Verification items for this drawing (mm, ordinates from the low corner). A direction names the side the tool comes from. Coordinates: 2 decimals unless noted, no trailing zeros. Write each loop counter-clockwise with the first axis right and the second up, starting at its lowest first coordinate (ties: lowest second). Pieces come first, ordered by that corner, then holes. Notation, with made-up numbers: M -34.5,88.25 L 10.5,88.25 A30 ccw 10.5,121.25 Z; hole C 54.25,41.5 d2. An arc over 180 degrees is marked long. Answer as CSV lines item,"result". Start each with the question number.
1) Section check D-D (x = 6). Record the cut outline in (y, z), and give its area (3 significant figures).
2) Draft check along X on the marked faces 1, 2 and 3. Enter one of: +X half, -X half, draft (parallel to the pull), parting line (faces both ways), or undercut.
3) Go/stop test with flat-tipped pins: pin 1 Ø1 at (x, z) = (12.5, 4) entering from -Y; pin 2 Ø3 at (y, z) = (17, 9.5) entering from -X; pin 3 Ø1.5 at (x, y) = (18, 25) entering from -Z (3 decimals). Record where each tip stops, or that it passes through.
4) Section check A-A (y = 19.05). Record the cut outline in (x, z) (1 decimal).
5) Material ranges on L1, parallel to Z at x = 22.5, y = 5; L2, parallel to X at y = 11, z = 2.5 (1 decimal); L3, parallel to X at y = 15, z = 8 (1 decimal), recorded low to high. Write a range as [from, to].
6) Access from +Z, -Z, +X, -X, +Y, -Y to the whole of each face (thin tool, end or side, straight path). Record for the marked faces 4, 5 and 6.
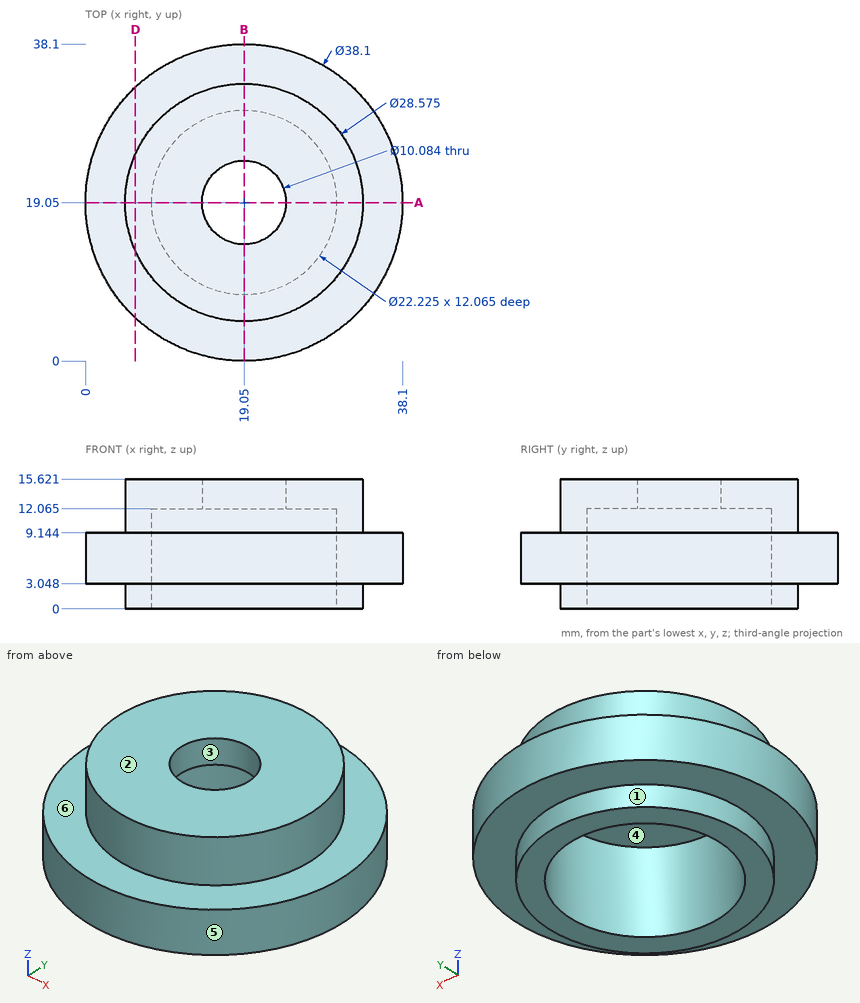
Results found:
1,outline,"M 5.17,3.05 L 13.23,3.05 L 13.23,0 L 24.87,0 L 24.87,3.05 L 32.93,3.05 L 32.93,9.14 L 24.87,9.14 L 24.87,15.62 L 13.23,15.62 L 13.23,9.14 L 5.17,9.14 Z"
1,area,"280 mm2"
2,face 1,"parting line"
2,face 2,"draft"
2,face 3,"undercut"
3,pin 1,"stops at y = 0.99"
3,pin 2,"stops at x = 0.01"
3,pin 3,"stops at z = 12.065"
4,outline,"M 0,3 L 4.8,3 L 4.8,0 L 7.9,0 L 7.9,12.1 L 14,12.1 L 14,15.6 L 4.8,15.6 L 4.8,9.1 L 0,9.1 Z; M 24.1,12.1 L 30.2,12.1 L 30.2,0 L 33.3,0 L 33.3,3 L 38.1,3 L 38.1,9.1 L 33.3,9.1 L 33.3,15.6 L 24.1,15.6 Z"
5,L1,"z = [3.05, 9.14]"
5,L2,"x = [7.2, 11.4], [26.7, 30.9]"
5,L3,"x = [0.4, 8.7], [29.4, 37.7]"
6,face 4,"-Z"
6,face 5,"+Z, -Z"
6,face 6,"+Z"
